Model file for the job. Use its own axes, mm. A direction names the side the tool comes from. Give positions to 0.01 mm unless a question says otherwise; leave off trailing zeros. Order: outer loops, then holes, each group sorted by start corner. A loop starts at its lowest first (then second) coordinate and runs counter-clockwise, first axis right, second up. Notation, with made-up numbers: (-1.75, 75) - (4.25, 75) arc R32 cw to (4.25, 113) - close; hole circle Ø9 at (-36.5, -34). An arc over 180 degrees is marked (long way). Return JSON: item names as keys, results as strings. Group by question number.
from build123d import *

# Parameters (mm, degrees)
BOSS_EXTRUDE1_START        = -25.4
BOSS_EXTRUDE1_DEPTH        = 25.4
BOSS_EXTRUDE2_DEPTH        = 4.7625
M6_5_CLEARANCE_HOLE1_D     = 7.1374
M6_5_CLEARANCE_HOLE1_DEPTH = 25.4
M6_5_CLEARANCE_HOLE2_D     = 7.1374
FILLET1_R                  = 3.175


with BuildPart() as part:
    # Boss-Extrude1: read off the stored shape, not the designer's step
    # Boss-Extrude1 outline → Boss-Extrude1 (new body)
    with BuildSketch(Plane(origin=(0, 0, 0), x_dir=(1, 0, 0), z_dir=(0, 1, 0)).offset(BOSS_EXTRUDE1_START)):
        with BuildLine():
            Line((-4.7625, -4.7625), (-4.7625, 0))
            Line((-4.7625, 0), (-50.8, 0))
            ThreePointArc((-50.8, 0), (-49.405096045, -3.367596045), (-46.0375, -4.7625))
            Line((-46.0375, -4.7625), (-4.7625, -4.7625))
        make_face()
    extrude(amount=BOSS_EXTRUDE1_DEPTH)

    # Sketch2 → Boss-Extrude2 (add)
    with BuildSketch(Plane(origin=(-4.7625, 0, 0), x_dir=(0, 0, -1), z_dir=(1, 0, 0))):
        with BuildLine():
            Line((0, 0), (0, -25.4))
            Line((0, -25.4), (-12.7, -25.4))
            ThreePointArc((-12.7, -25.4), (-25.4, -12.7), (-12.7, 0))
            Line((-12.7, 0), (0, 0))
        make_face()
    extrude(amount=BOSS_EXTRUDE2_DEPTH)

    # M6.5 Clearance Hole1
    with Locations(Plane(origin=(0, 0, 0), x_dir=(-1, 0, 0), z_dir=(0, 0, -1))):
        with Locations((38.1, -12.7), (12.7, -12.7)):
            Hole(M6_5_CLEARANCE_HOLE1_D / 2, depth=M6_5_CLEARANCE_HOLE1_DEPTH)

    # M6.5 Clearance Hole2 (through all)
    with Locations(Plane.ZY.offset(4.7625)):
        with Locations((12.7, -12.7)):
            Hole(M6_5_CLEARANCE_HOLE2_D / 2)

    # Fillet1
    fillet1_edges = [part.edges().sort_by_distance(p)[0] for p in [
        (-4.7625, -12.7, 4.7625),
    ]]
    fillet(fillet1_edges, radius=FILLET1_R)


solid = part.part
(1) Slice it at C-C (z = 10.75). Give the cut face in (x, y).
(2) Drop flat-ended pins along their axis: pin 1 Ø12 at (x, y) = (-7.5, -7.5) entering from -Z; pin 2 Ø10 at (y, z) = (-15.5, 20) entering from -X; pin 3 Ø8 at (x, y) = (-38.1, -12.7) entering from +Z. Give the stop position or say it passes through.
(3) Drill centre lines: L1, parallel to Y at x = -38.1, z = 1.8; L2, parallel to X at y = -22, z = 11.75; L3, parallel to Z at x = -29, y = -7.5. Where is each one in solid material? Low to high.
(4) Slice it at A-A (x = -38.1). Give the cut face in (y, z).
(5) Pull direction X, two halves, no side cores. Call faces 1 (the face through (-2.348, -12.543, 16.265)), 2 (the face through (-5.717, -12.522, 5.668)), 3 (the face through (-34.696, -11.628, 2.415)), 4 (the face through (-16.265, -12.543, 2.415)): released by +X, released by -X, zero draft, split by the parting line, or undercut.
(6) Slice it at B-B (y = -12.7). State how many separate pieces and enclosed holes the cut face has, and give its area (3 significant figures).
(7) 3-axis set-ups, long thin cutter, end or side, ignore diameter. For faces 5 (the face through (-27, -13, 4.762)), 6 (the face through (-2.415, -12.979, 25.397)): which of +Z, -Z, +X, -X, +Y, -Y reach the whole face in a straight line?
(8) Slice it at D-D (z = 2.75). Give the cut face in (x, y), and give its area (3 significant figures).
Result set:
{
 "1": {"outline": "(-4.76, -25.4) - (0, -25.4) - (0, -15.69) - (-4.76, -15.69) - close; (-4.76, -9.71) - (0, -9.71) - (0, 0) - (-4.76, 0) - close"},
 "2": {"pin 1": "stops at z = 0", "pin 2": "stops at x = -4.76", "pin 3": "stops at z = 4.76"},
 "3": {"L1": "y = -25.4 to -16.27, -9.13 to 0", "L2": "x = -4.76 to 0", "L3": "z = 0 to 4.76"},
 "4": {"outline": "(-25.4, 0) - (-16.27, 0) - (-16.27, 4.76) - (-25.4, 4.76) - close; (-9.13, 0) - (0, 0) - (0, 4.76) - (-9.13, 4.76) - close"},
 "5": {"face 1": "zero draft", "face 2": "released by -X", "face 3": "undercut", "face 4": "undercut"},
 "6": {"separate pieces": "4", "enclosed holes": "0", "area": "236 mm²"},
 "7": {"face 5": "+Z, -X, +Y, -Y", "face 6": "+Z, +X, -X"},
 "8": {"outline": "(-49.93, -25.4) - (0, -25.4) - (0, 0) - (-49.93, 0) - close; hole circle Ø7.14 at (-38.1, -12.7); hole circle Ø7.14 at (-12.7, -12.7)", "area": "1,190 mm²"}
}
